Geometry check sheet. Reference: the model listing, model coordinates, mm. Face numbers are marked on the shaded views. Coordinates: 2 decimals unless noted, no trailing zeros. Write each loop counter-clockwise with the first axis right and the second up, starting at its lowest first coordinate (ties: lowest second). Pieces come first, ordered by that corner, then holes. Notation, with made-up numbers: (48, -36.75) -> (92, -36.75) arc R16 ccw to (92, -7.75) -> close; hole circle Ø4 at (32, 54). An arc over 180 degrees is marked (long way). Answer in a Markdown table with one row per item. Add a question column.
Q1. Thickness scan on line 1 (X direction, y = 51.5, z = 151); line 2 (Y direction, x = 75, z = 145); line 3 (Y direction, x = 89.5, z = 135.5). Record the ranges inside material, lowest first.
Q2. Gauge pin test, flat ends, axial feed: P1, Ø1.5, axis at x = 69, y = 40.5, coming from the -Z side; P2, Ø2, axis at x = 77.5, y = 49.5, coming from the -Z side; P3, Ø12, axis at x = 59, y = 27.5, coming from the +Z side; P4, Ø5, axis at y = 33, z = 128.5, coming from the -X side. Record the tip position at first contact, or that the pin passes through.
Q3. Section check D-D, the plane z = 138.5. Record the boundary of the cut face in (x, y).
Q4. Section check C-C, the plane x = 63. Record the boundary of the cut face in (y, z).
Q5. Release check for a two-part mould opening along Z. For the marked faces 1, 2, 3 and 4 record: pulls with the +Z half, pulls with the -Z half, needs draft (parallel to the pull), parting line crosses it, or undercut.
Q6. Section check B-B, the plane x = 75. Record the boundary of the cut face in (y, z), and give its area (3 significant figures).
Q7. Section check A-A, the plane x = 58. Record the boundary of the cut face in (y, z).
```python
from build123d import *

# Parameters (mm, degrees)
SKETCH1_W           = 37
SKETCH1_H           = 39
SKETCH1_R           = 1.5
BOSS_EXTRUDE1_DEPTH = 7.5
SKETCH2_R           = 2
CUT_EXTRUDE1_DEPTH  = 177.665153947


with BuildPart() as part:
    # Sketch1 → Boss-Extrude1 (new body)
    with BuildSketch(Plane(origin=(0, -53.862394692, 53.862394692), x_dir=(1, 0, 0), z_dir=(0, 0.7071067811865502, -0.7071067811865449))):
        with Locations((73.844609768, -127.312236852)):
            Rectangle(SKETCH1_W, SKETCH1_H)
        with Locations(Location((88.844609768, -143.812236852, 0), (0, 0, 270))):
            Circle(SKETCH1_R, mode=Mode.SUBTRACT)
        with Locations(Location((58.844609768, -143.812236852, 0), (0, 0, 270))):
            Circle(SKETCH1_R, mode=Mode.SUBTRACT)
        with Locations(Location((58.844609768, -110.812236852, 0), (0, 0, 270))):
            Circle(SKETCH1_R, mode=Mode.SUBTRACT)
        with Locations(Location((88.844609768, -110.812236852, 0), (0, 0, 270))):
            Circle(SKETCH1_R, mode=Mode.SUBTRACT)
    extrude(amount=BOSS_EXTRUDE1_DEPTH)

    # Sketch2 → Cut-Extrude1 (cut, through all)
    with BuildSketch(Plane(origin=(0, -48.559093833, 48.559093833), x_dir=(1, 0, 0), z_dir=(0, 0.7071067811865502, -0.7071067811865449))):
        with Locations(Location((73.844609768, -131.312236852, 0), (0, 0, 270))):
            Circle(SKETCH2_R)
    extrude(amount=-CUT_EXTRUDE1_DEPTH, mode=Mode.SUBTRACT)


solid = part.part
```
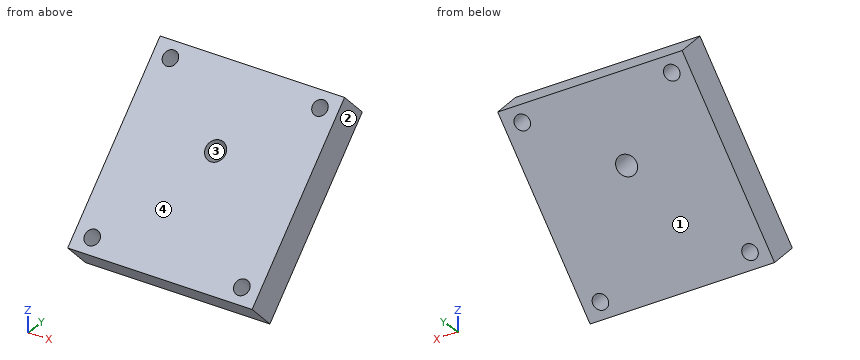
Calculated:
| question | item | result |
|---|---|---|
| 1 | line 1 | x = 55.34 to 57.48, 60.21 to 87.48, 90.21 to 92.34 |
| 1 | line 2 | y = 37.28 to 38.39, 43.01 to 47.88 |
| 1 | line 3 | y = 27.78 to 38.38 |
| 2 | P1 | stops at z = 136.87 |
| 2 | P2 | stops at z = 145.62 |
| 2 | P3 | stops at z = 141.22 |
| 2 | P4 | stops at x = 55.34 |
| 3 | outline | (55.34, 30.78) -> (92.34, 30.78) -> (92.34, 41.38) -> (55.34, 41.38) -> close |
| 4 | outline | (22.37, 130.1) -> (27.68, 124.79) -> (55.25, 152.37) -> (49.95, 157.67) -> close |
| 5 | face 1 | pulls with the -Z half |
| 5 | face 2 | needs draft |
| 5 | face 3 | undercut |
| 5 | face 4 | pulls with the +Z half |
| 6 | outline | (22.37, 130.1) -> (27.68, 124.79) -> (43.14, 140.26) -> (37.84, 145.56) -> close; (40.14, 147.87) -> (45.45, 142.57) -> (55.25, 152.37) -> (49.95, 157.67) -> close |
| 6 | area | 268 mm² |
| 7 | outline | (22.37, 130.1) -> (27.68, 124.79) -> (28.92, 126.04) -> (23.62, 131.34) -> close; (25.37, 133.1) -> (30.67, 127.79) -> (52.25, 149.37) -> (46.95, 154.68) -> close; (48.7, 156.43) -> (54.01, 151.13) -> (55.25, 152.37) -> (49.95, 157.67) -> close |
